```python
from build123d import *

# Parameters (mm, degrees)
PAD_DEPTH       = 56.5
SKETCH049_W     = 9.963656
SKETCH049_H     = 4.853651
SKETCH049_W_2   = 14.419268
SKETCH049_H_2   = 9.8
SKETCH049_W_3   = 14.165799
SKETCH049_W_4   = 9.249737
SKETCH049_H_3   = 3.2
POCKET033_DEPTH = 10
SKETCH050_R     = 1.4
POCKET034_DEPTH = 113.001
SKETCH051_R     = 1.75
POCKET035_DEPTH = 7
SKETCH052_R     = 1.75
POCKET036_DEPTH = 7
SKETCH053_R     = 1.9
POCKET037_DEPTH = 10
FILLET_R        = 1


with BuildPart() as part:
    # Sketch041 → Pad (new body, symmetric)
    with BuildSketch(Plane.YZ):
        Polygon((-11, 0), (-11, 3), (-6, 8), (-6, 66), (0, 66), (0, 8), (5, 3), (5, 0), (0, 0), align=None)
    extrude(amount=PAD_DEPTH, both=True)

    # Sketch049 (on Face4 of Pad) → Pocket033 (cut)
    with BuildSketch(Plane(origin=(0, 0, 66), x_dir=(0, -1, 0), z_dir=(0, 0, 1))):
        with Locations((1.82395, 59.0693)):
            Rectangle(SKETCH049_W, SKETCH049_H)
        with Locations((2.618054, 46.004022)):
            Rectangle(SKETCH049_W_2, SKETCH049_H_2)
        with Locations((0.916195, -45.939361)):
            Rectangle(SKETCH049_W_3, SKETCH049_H_2)
        with Locations((2.129443, -58.515822)):
            Rectangle(SKETCH049_W_4, SKETCH049_H_3)
    extrude(amount=-POCKET033_DEPTH, mode=Mode.SUBTRACT)

    # Sketch050 (on Face5 of Pocket033) → Pocket034 (cut, through all)
    with BuildSketch(Plane.YZ.offset(56.5)):
        with Locations((-3, 63)):
            Circle(SKETCH050_R)
    extrude(amount=-POCKET034_DEPTH, mode=Mode.SUBTRACT)

    # Sketch051 (on Face5 of Pocket034) → Pocket035 (cut)
    with BuildSketch(Plane.YZ.offset(56.5)):
        with Locations((-2.965743, 62.998383)):
            Circle(SKETCH051_R)
    extrude(amount=-POCKET035_DEPTH, mode=Mode.SUBTRACT)

    # Sketch052 (on Face4 of Pocket035) → Pocket036 (cut)
    with BuildSketch(Plane(origin=(-56.5, 0, 0), x_dir=(0, 1, 0), z_dir=(-1, 0, 0))):
        with Locations((-3.013862, -62.999382)):
            Circle(SKETCH052_R)
    extrude(amount=-POCKET036_DEPTH, mode=Mode.SUBTRACT)

    # Sketch053 (on Face2 of Pocket036) → Pocket037 (cut)
    with BuildSketch(Plane.YX):
        with Locations((-3, 40)):
            Circle(SKETCH053_R)
        with Locations((-3, -40)):
            Circle(SKETCH053_R)
    extrude(amount=-POCKET037_DEPTH, mode=Mode.SUBTRACT)

    # Fillet
    fillet_edges = [part.edges().sort_by_distance(p)[0] for p in [
        (0.03233, -6, 66),
        (53.702011, -6, 66),
        (-53.66968, -6, 66),
    ]]
    fillet(fillet_edges, radius=FILLET_R)


with BuildPart() as part_1:
    # Body placement: moved
    add(part.part.moved(Location((-1.5, 0, 0))))


solid = part_1.part
```
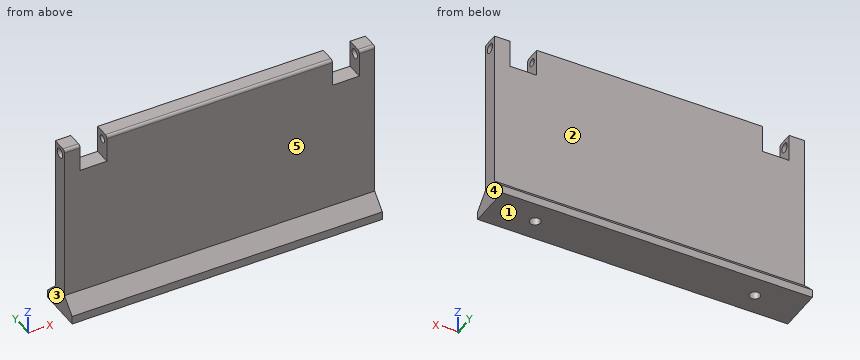
Work out the finished part from the listing and answer in its coordinate system (mm). Face numbers are marked on the shaded views. A direction names the side the tool comes from. Round coordinates to 2 decimals unless told otherwise and drop trailing zeros. Loops run counter-clockwise (first coordinate to the right, second up) from the corner with the lowest first, then second, coordinate; pieces in that order, holes last. Notation, with made-up numbers: (-2.5, 89) -> (22.5, 89) arc R32 cw to (22.5, 121) -> close; hole circle Ø8 at (68, -4). An arc over 180 degrees is marked (long way). Write each question's results on one line, items separated by ' | '. Start each with the question number.
1. Section A-A (x = 38.5) is taken. Determine the outline of the cut face in (y, z).
2. Section D-D (z = 37.5) is taken. Determine the outline of the cut face in (x, y).
3. Find the intervals of material crossed by probe 1 along Y at (x, z) = (19, 27); probe 2 along Y at (x, z) = (-41, 3); probe 3 along Z at (x, y) = (-4.5, -1.75), in increasing order. Write a range as from..to.
4. Given pin 1 Ø1.1 at (x, y) = (-42, -3) entering from -Z; pin 2 Ø6.5 at (x, y) = (-46.5, -4.5) entering from +Z; pin 3 Ø3 at (x, z) = (-13, 7) entering from -Y; pin 4 Ø3 at (y, z) = (-1.5, 63.5) entering from -X, each flat-ended and moving along its own axis, determine where each tip first touches the part or whether it passes through.
5. Section C-C (x = 22) is taken. Determine the outline of the cut face in (y, z), plus the area to 3 significant figures.
6. Section B-B (y = -3) is taken. State how many separate pieces and enclosed holes the cut face has, plus the area to 3 significant figures.
7. For a pull along X with two mould halves and no side action, classify the marked faces 3, 4 and 5 as +X half, -X half, draft (parallel to the pull), parting line (faces both ways), or undercut.
8. A tool of negligible diameter and unlimited length cuts with its end or side. For the marked faces 1 and 2, from which of +Z, -Z, +X, -X, +Y, -Y can it reach the whole face along a straight path? Write none if from no direction.
Evaluation:
1) outline: (-11, 0) -> (-4.9, 0) -> (-4.9, 10) -> (-1.1, 10) -> (-1.1, 0) -> (5, 0) -> (5, 3) -> (0, 8) -> (0, 66) -> (-5, 66) arc R1 ccw to (-6, 65) -> (-6, 8) -> (-11, 3) -> close; hole circle Ø2.8 at (-3, 63)
2) outline: (-58, -6) -> (55, -6) -> (55, 0) -> (-58, 0) -> close
3) probe 1: y = -6..0 | probe 2: y = -11..-4.83, -1.17..5 | probe 3: z = 0..62.37, 63.63..66
4) pin 1: stops at z = 10 | pin 2: stops at z = 56 | pin 3: stops at y = -8.5 | pin 4: stops at x = -58
5) outline: (-11, 0) -> (5, 0) -> (5, 3) -> (0, 8) -> (0, 66) -> (-5, 66) arc R1 ccw to (-6, 65) -> (-6, 8) -> (-11, 3) -> close; hole circle Ø2.8 at (-3, 63) | area: 445 mm2
6) separate pieces: 4 | enclosed holes: 0 | area: 6,920 mm2
7) face 3: -X half | face 4: +X half | face 5: draft
8) face 1: -Z, +X, -X, +Y, -Y | face 2: +Z, +X, -X, +Y
